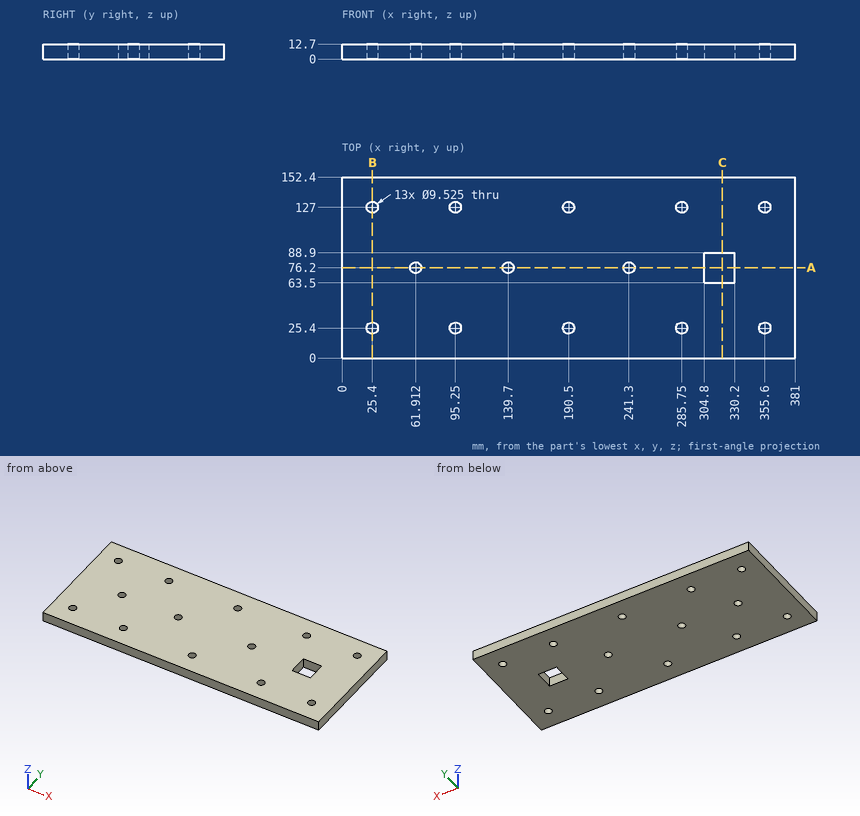
Geometry check sheet. Reference: drawing and pictorial views, mm from the part's lowest x, y, z. Round coordinates to 2 decimals unless told otherwise and drop trailing zeros. Loops run counter-clockwise (first coordinate to the right, second up) from the corner with the lowest first, then second, coordinate; pieces in that order, holes last.
1. Sectioned sample at A-A on y = 76.2. Give the number of separate pieces and of enclosed holes in the cut face, and give its area (3 significant figures).
2. Gauge pin test, flat ends, axial feed: pin 1 Ø11 at (x, y) = (61.91, 76.2) entering from +Z; pin 2 Ø5.5 at (x, y) = (241.3, 76.2) entering from +Z. Record the tip position at first contact, or that the pin passes through.
3. Sectioned sample at C-C on x = 320. Record the boundary of the cut face in (y, z), and give its area (3 significant figures).
4. Sectioned sample at B-B on x = 25.4. Record the boundary of the cut face in (y, z).
5. Scan lines: probe 1 along Y at (x, z) = (95.25, 3.5); probe 2 along X at (y, z) = (69.5, 11); probe 3 along Y at (x, z) = (139.7, 3.75). Record each from-to range of solid material in increasing order.
Recorded:
1. separate pieces: 5
1. enclosed holes: 0
1. area: 4,150 mm2
2. pin 1: stops at z = 12.7
2. pin 2: passes through
3. outline: (0, 0) - (63.5, 0) - (63.5, 12.7) - (0, 12.7) - close; (88.9, 0) - (152.4, 0) - (152.4, 12.7) - (88.9, 12.7) - close
3. area: 1,610 mm2
4. outline: (0, 0) - (20.64, 0) - (20.64, 12.7) - (0, 12.7) - close; (30.16, 0) - (122.24, 0) - (122.24, 12.7) - (30.16, 12.7) - close; (131.76, 0) - (152.4, 0) - (152.4, 12.7) - (131.76, 12.7) - close
5. probe 1: y = 0 to 20.64, 30.16 to 122.24, 131.76 to 152.4
5. probe 2: x = 0 to 304.8, 330.2 to 381
5. probe 3: y = 0 to 71.44, 80.96 to 152.4
